Source: CAD feature listing. Evaluate the final solid. Frame: model axes, mm. Face numbers are marked on the shaded views. A direction names the side the tool comes from. Give positions to 0.01 mm unless a question says otherwise; leave off trailing zeros. Order: outer loops, then holes, each group sorted by start corner. A loop starts at its lowest first (then second) coordinate and runs counter-clockwise, first axis right, second up.
1) Section A-A, the plane z = 8.25. Return loops of the section in (x, y).
2) Section B-B, the plane y = -1.5. Return loops of the section in (x, z).
3) First-contact query: P1, Ø3, axis at y = -6, z = 2.5, coming from the -X side; P2, Ø5, axis at x = 6, y = -7, coming from the -Z side. Flat tips, straight axial feed; report the tip coordinate or a pass-through.
4) Draft query along X for the marked faces 3, 4, 5 and 6. Return one class per face: released by +X, released by -X, zero draft, split by the parting line, or undercut.
5) Access query for the marked faces 1 and 2. Directions: +Z, -Z, +X, -X, +Y, -Y. A direction counts if a zero-diameter tool reaches every point of the face in a straight line with its end or side. Return the directions, or none.
6) Section C-C, the plane z = -3. Return loops of the section in (x, y).
7) Material intervals for line 1 (Z direction, x = 1, y = -5.5); line 2 (X direction, y = -5.75, z = 4); line 3 (X direction, y = -7.25, z = -0.25), sorted ascending.
8) Section D-D, the plane x = 6. Return loops of the section in (y, z).
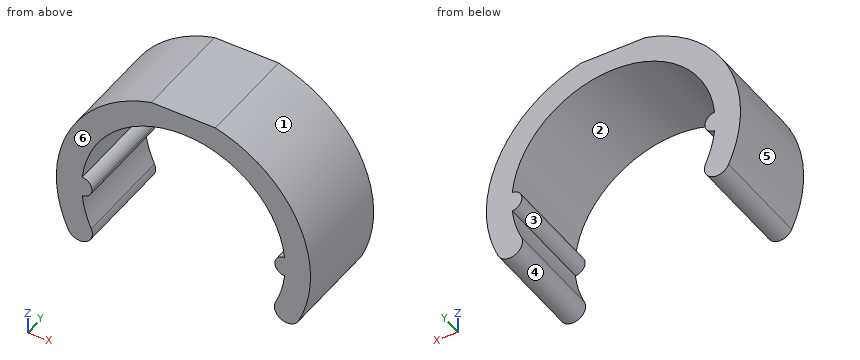
```python
from build123d import *

# Parameters (mm, degrees)
F1_DEPTH = 10


with BuildPart() as f1:
    # F0 (on Front) → F1 (new body)
    with BuildSketch(Plane.XZ):
        with BuildLine():
            ThreePointArc((-9.95, 0.9987492178), (-10, 0), (-9.95, -0.9987492178))
            ThreePointArc((-9.95, -0.9987492178), (-9.2754311627, -0.6892024376), (-9, 0))
            ThreePointArc((-9, 0), (-9.2754311627, 0.6892024376), (-9.95, 0.9987492178))
        make_face()
        with BuildLine():
            ThreePointArc((9.95, -0.9987492178), (10, 0), (9.95, 0.9987492178))
            ThreePointArc((9.95, 0.9987492178), (9, 0), (9.95, -0.9987492178))
        make_face()
        with BuildLine():
            ThreePointArc((-9.95, 0.9987492178), (-11, 0), (-9.95, -0.9987492178))
            ThreePointArc((-9.95, -0.9987492178), (-10, 0), (-9.95, 0.9987492178))
        make_face()
        with BuildLine():
            ThreePointArc((11, 0), (10.6892024376, 0.7245688373), (9.95, 0.9987492178))
            ThreePointArc((9.95, 0.9987492178), (10, 0), (9.95, -0.9987492178))
            ThreePointArc((9.95, -0.9987492178), (10.6892024376, -0.7245688373), (11, 0))
        make_face()
        with BuildLine():
            ThreePointArc((-11.328847338, -5.2827282718), (-9.667689777, -5.8873401784), (-9.0630778704, -4.2261826174))
            ThreePointArc((-9.0630778704, -4.2261826174), (-9.6425289273, -2.6498369547), (-9.95, -0.9987492178))
            ThreePointArc((-9.95, -0.9987492178), (-11, 0), (-9.95, 0.9987492178))
            ThreePointArc((-9.95, 0.9987492178), (0, 10), (9.95, 0.9987492178))
            ThreePointArc((9.95, 0.9987492178), (10.6892024376, 0.7245688373), (11, 0))
            ThreePointArc((11, 0), (10.6892024376, -0.7245688373), (9.95, -0.9987492178))
            ThreePointArc((9.95, -0.9987492178), (9.6425289273, -2.6498369547), (9.0630778704, -4.2261826174))
            ThreePointArc((9.0630778704, -4.2261826174), (9.667689777, -5.8873401784), (11.328847338, -5.2827282718))
            ThreePointArc((11.328847338, -5.2827282718), (11.3110273164, 5.3207763577), (3.1539999452, 12.0955481209))
            Line((3.1539999452, 12.0955481209), (-3.1539999452, 12.0955481209))
            ThreePointArc((-3.1539999452, 12.0955481209), (-11.3110273164, 5.3207763577), (-11.328847338, -5.2827282718))
        make_face()
    extrude(amount=F1_DEPTH)


solid = f1.part
```
From the geometry:
1. outline: (-9.39, -10) - (-5.65, -10) - (-5.65, 0) - (-9.39, 0) - close; (5.65, -10) - (9.39, -10) - (9.39, 0) - (5.65, 0) - close
2. outline: (-11.33, -5.28) arc R1.25 ccw to (-9.06, -4.23) arc R10 cw to (-9.95, -1) arc R1 ccw to (-9.95, 1) arc R10 cw to (9.95, 1) arc R1 ccw to (9.95, -1) arc R10 cw to (9.06, -4.23) arc R1.25 ccw to (11.33, -5.28) arc R12.5 ccw to (3.15, 12.1) - (-3.15, 12.1) arc R12.5 ccw to start
3. P1: stops at x = -12.46
3. P2: stops at z = 5.27
4. face 3: undercut
4. face 4: undercut
4. face 5: released by -X
4. face 6: zero draft
5. face 1: +X, +Y, -Y
5. face 2: +Y, -Y
6. outline: (-12.13, -10) - (-9.54, -10) - (-9.54, 0) - (-12.13, 0) - close; (9.54, -10) - (12.13, -10) - (12.13, 0) - (9.54, 0) - close
7. line 1: z = 9.95 to 12.1
7. line 2: x = -11.84 to -9.17, 9.17 to 11.84
7. line 3: x = -12.5 to -9.03, 9.03 to 12.5
8. outline: (-10, 8) - (0, 8) - (0, 10.97) - (-10, 10.97) - close
